Input: part model. Units: mm. Frame: model coordinates. A direction names the side the tool comes from. Round coordinates to 2 decimals unless told otherwise and drop trailing zeros. Loops run counter-clockwise (first coordinate to the right, second up) from the corner with the lowest first, then second, coordinate; pieces in that order, holes last.
1) Access query for faces 1 (the face through (4, 3, 12.923)), 2 (the face through (1.45, 4.56, -6.02)). Directions: +Z, -Z, +X, -X, +Y, -Y. A direction counts if a zero-diameter tool reaches every point of the face in a straight line with its end or side. Return the directions, or none.
2) Ray query, line 1 along Y through (x, z) = (4.5, -4); line 2 along Z through (x, y) = (5.75, 4.75); line 3 along Z through (x, y) = (8.25, 2.75). Return the intervals inside material, ascending.
3) Section A-A, the plane x = 0.75. Return loops of the section in (y, z), and give its area (3 significant figures).
4) Section B-B, the plane z = 6.5. Return loops of the section in (x, y).
5) Section D-D, the plane y = 9. Return loops of the section in (x, z), and give its area (3 significant figures).
6) Section C-C, the plane y = -2.25. Return loops of the section in (x, z).
7) Draft query along Y for faces 3 (the face through (4.764, 3.809, -0.438)), 4 (the face through (4, -3.199, -2)), 5 (the face through (4.56, 8.09, 11.12)), 6 (the face through (0, 3, 2)). Return one class per face: pulls with the +Y half, pulls with the -Y half, needs draft (parallel to the pull), parting line crosses it, or undercut.
from build123d import *

# Parameters (mm, degrees)
F0_W     = 13
F0_H     = 23
F1_DEPTH = 9
F2_R     = 6
F4_DEPTH = 9.001
F6_D     = 6.6
F6_DEPTH = 8
F6_TIP   = 1.9828400428


with BuildPart() as f1:
    # F0 (on Right) → F1 (new body)
    with BuildSketch(Plane.YZ):
        with Locations((3.3005997539, 1.423231575)):
            Rectangle(F0_W, F0_H)
    extrude(amount=F1_DEPTH)

    # F2
    f2_edges = [f1.edges().sort_by_distance(p)[0] for p in [
        (4.5, -3.1994, 12.923232),
        (4.5, 9.8006, 12.923232),
    ]]
    fillet(f2_edges, radius=F2_R)

    # F3 (on face) → F4 (cut, through all)
    with BuildSketch(Plane.YZ.offset(9)):
        with BuildLine():
            ThreePointArc((5.3005997539, 4.923231575), (4.7148133162, 6.3374451374), (3.3005997539, 6.923231575))
            Line((3.3005997539, 6.923231575), (3.3005997539, 2.923231575))
            ThreePointArc((3.3005997539, 2.923231575), (4.7148133162, 3.5090180127), (5.3005997539, 4.923231575))
        make_face()
        with BuildLine():
            Line((3.3005997539, 2.923231575), (3.3005997539, 6.923231575))
            ThreePointArc((3.3005997539, 6.923231575), (1.3005997539, 4.923231575), (3.3005997539, 2.923231575))
        make_face()
    extrude(amount=-F4_DEPTH, mode=Mode.SUBTRACT)

    # F6
    with Locations(Plane(origin=(0, 0, -10.076768425), x_dir=(1, 0, 0), z_dir=(0, 0, -1))):
        with Locations((4.5, -3.3005997539)):
            Hole(F6_D / 2, depth=F6_DEPTH)
            with Locations((0, 0, -(F6_DEPTH + F6_TIP / 2))):  # 118° drill point
                Cone(0, F6_D / 2, F6_TIP, mode=Mode.SUBTRACT)


solid = f1.part
Final values:
1. face 1: +Z, +X, -X, +Y, -Y
1. face 2: -Z
2. line 1: y = -3.2 to 0, 6.6 to 9.8
2. line 2: z = -1.24 to 3.55, 6.3 to 12.85
2. line 3: z = -10.08 to 3, 6.85 to 12.92
3. outline: (-3.2, -10.08) - (9.8, -10.08) - (9.8, 6.92) arc R6 ccw to (3.8, 12.92) - (2.8, 12.92) arc R6 ccw to (-3.2, 6.92) - close; hole circle Ø4 at (3.3, 4.92)
3. area: 271 mm2
4. outline: (0, -3.2) - (9, -3.2) - (9, 2.07) - (0, 2.07) - close; (0, 4.53) - (9, 4.53) - (9, 9.8) - (0, 9.8) - close
5. outline: (0, -10.08) - (9, -10.08) - (9, 9.92) - (0, 9.92) - close
5. area: 180 mm2
6. outline: (0, -10.08) - (9, -10.08) - (9, 10.16) - (0, 10.16) - close
7. face 3: undercut
7. face 4: pulls with the -Y half
7. face 5: pulls with the +Y half
7. face 6: needs draft
